Could you check a few things on this model? Use its own coordinates, in mm. A direction names the side the tool comes from. Round coordinates to 2 decimals unless told otherwise and drop trailing zeros. Write each loop counter-clockwise with the first axis right and the second up, starting at its lowest first coordinate (ties: lowest second). Pieces come first, ordered by that corner, then holes. Notation, with made-up numbers: (-27, 48.5) - (-18, 48.5) arc R11 cw to (-18, 68.5) - close; hole circle Ø4 at (4.5, 73.5). An arc over 180 degrees is marked (long way). Put each result on its own line as item: value.
from build123d import *

# Parameters (mm, degrees)
F0_W     = 22
F0_H     = 22
F0_W_2   = 19.05
F0_H_2   = 19.05
F1_DEPTH = 12.5
F2_R     = 2.38125
F3_DEPTH = 3
F4_R     = 2.38125
F5_DEPTH = 3
F6_R     = 2.38125
F7_DEPTH = 3
F8_R     = 2.4003
F9_DEPTH = 3
F10_R    = 1


# Not quite as in the source:
# - a feature names something its author has since deleted; it is built from what else it names


with BuildPart() as f1:
    # F0 (on Top) → F1 (new body, symmetric)
    with BuildSketch(Plane.XY):
        Rectangle(F0_W, F0_H)
        Rectangle(F0_W_2, F0_H_2, mode=Mode.SUBTRACT)
    extrude(amount=F1_DEPTH, both=True)

    # F2 (on Front) → F3 (join)
    with BuildSketch(Plane.XZ):
        with BuildLine():
            Line((-11, -12.5), (-11, 12.5))
            Line((-11, 12.5), (-19.6206896552, 3.4482758621))
            ThreePointArc((-19.6206896552, 3.4482758621), (-21, 0), (-19.6206896552, -3.4482758621))
            Line((-19.6206896552, -3.4482758621), (-11, -12.5))
        make_face()
        with Locations((-16, 0)):
            Circle(F2_R, mode=Mode.SUBTRACT)
    extrude(amount=F3_DEPTH)

    # F4 (on Right) → F5 (join)
    with BuildSketch(Plane.YZ):
        with BuildLine():
            Line((-11, 12.5), (-19.6206896552, 3.4482758621))
            ThreePointArc((-19.6206896552, 3.4482758621), (-21, 0), (-19.6206896552, -3.4482758621))
            Line((-19.6206896552, -3.4482758621), (-11, -12.5))
            Line((-11, -12.5), (-11, 12.5))
        make_face()
        with Locations((-16, 0)):
            Circle(F4_R, mode=Mode.SUBTRACT)
    extrude(amount=F5_DEPTH)

    # F6 (on Front) → F7 (join)
    with BuildSketch(Plane.XZ):
        with BuildLine():
            Line((11, -12.5), (19.6206896552, -3.4482758621))
            ThreePointArc((19.6206896552, -3.4482758621), (21, 0), (19.6206896552, 3.4482758621))
            Line((19.6206896552, 3.4482758621), (11, 12.5))
            Line((11, 12.5), (11, -12.5))
        make_face()
        with Locations((16, 0)):
            Circle(F6_R, mode=Mode.SUBTRACT)
    extrude(amount=-F7_DEPTH)

    # F8 (on Right) → F9 (join)
    with BuildSketch(Plane.YZ):
        with BuildLine():
            ThreePointArc((19.6206896552, -3.4482758621), (21, 0), (19.6206896552, 3.4482758621))
            Line((19.6206896552, 3.4482758621), (11, 12.5))
            Line((11, 12.5), (11, -12.5))
            Line((11, -12.5), (19.6206896552, -3.4482758621))
        make_face()
        with Locations((16, 0)):
            Circle(F8_R, mode=Mode.SUBTRACT)
    extrude(amount=-F9_DEPTH)

    # F10
    f10_edges = [f1.edges().sort_by_distance(p)[0] for p in [
        (-11, -3, 0),
        (0, -11, 0),
        (3, -11, 0),
        (-11, 0, 0),
        (11, 0, 0),
        (11, 3, 0),
        (0, 11, 0),
        (-3, 11, 0),
    ]]
    fillet(f10_edges, radius=F10_R)


solid = f1.part
(1) I'm going to push flat-ended pins straight in: pin 1 (5.5 mm diameter, centred on x = -16, z = 0, fed in from +Y); pin 2 (5.5 mm diameter, centred on x = 9, z = 4, fed in from -Y); pin 3 (4 mm diameter, centred on x = 15, z = 3.5, fed in from +Y); pin 4 (12 mm diameter, centred on x = 16, y = 11.5, fed in from -Z). Where does each tip first touch, or does it pass through?
Values found:
pin 1: stops at y = 0
pin 2: stops at y = -11
pin 3: stops at y = 3
pin 4: stops at z = -12.5
(2) If we mould it in two halves opening along Z, with no side actions, what happens to faces 4 (the face through (15.25, 1.46, -8.04)), 5 (the face through (-8, 11, 0)), 6 (the face through (-1.48, 14.23, 1.62))? For each: pulls with the +Z half, pulls with the -Z half, needs draft (parallel to the pull), parting line crosses it, or undercut.
Values found:
face 4: pulls with the -Z half
face 5: needs draft
face 6: undercut
(3) Please list where these lines run through material, in increasing order: probe 1 along X at (y, z) = (-9, -10.75) (3 decimals); probe 2 along X at (y, z) = (12.5, 4). Write a range as from..to.
Values found:
probe 1: x = -11..-9.525, 9.525..11
probe 2: x = -3..0
(4) Imagine slicing it at B-B, the plane y = 16. List the corners of the cut face in (x, z) for me.
Values found:
outline: (-3, -7.25) - (0, -7.25) - (0, -2.4) - (-3, -2.4) - close; (-3, 2.4) - (0, 2.4) - (0, 7.25) - (-3, 7.25) - close
(5) Imagine slicing it at C-C, the plane x = 16. List the corners of the cut face in (y, z) for me.
Values found:
outline: (0, -7.25) - (3, -7.25) - (3, -2.38) - (0, -2.38) - close; (0, 2.38) - (3, 2.38) - (3, 7.25) - (0, 7.25) - close
(6) Imagine slicing it at A-A, the plane y = 2. List the corners of the cut face in (x, z) for me (1 decimal).
Values found:
outline: (-11, -12.5) - (-9.5, -12.5) - (-9.5, 12.5) - (-11, 12.5) - close; (9.5, -12.5) - (11, -12.5) - (19.6, -3.4) arc R5 ccw to (19.6, 3.4) - (11, 12.5) - (9.5, 12.5) - close; hole circle Ø4.8 at (16, 0)
(7) For faces 1 (the face through (-11, 6, 0)), 2 (the face through (-10, 0, -12.5)), 3 (the face through (3, -14.6, -2.4)), which set-ups out of +Z, -Z, +X, -X, +Y, -Y let a thin tool reach every point of the face, with its end or its side?
Values found:
face 1: +Z, -Z, -X, +Y
face 2: -Z, +X, -X, +Y, -Y
face 3: +Z, -Z, +X, -Y
